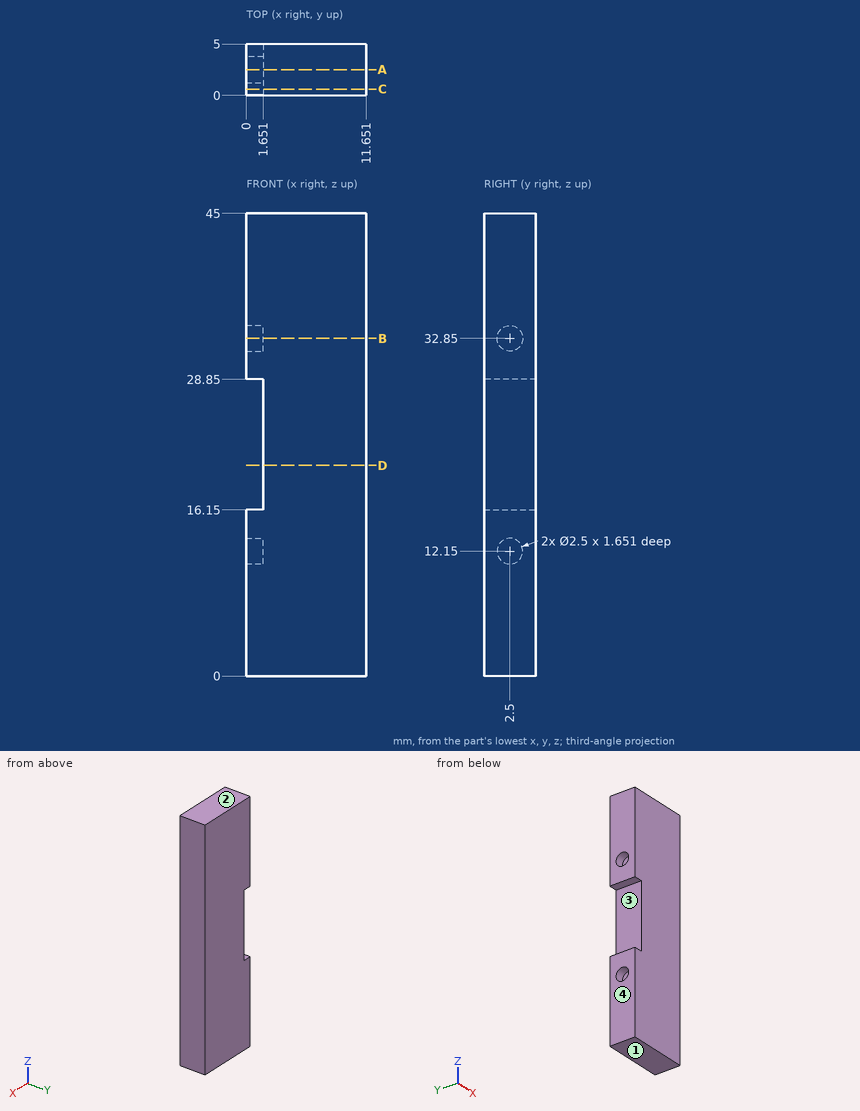
The drawing under review shows one solid part. Ordinate dimensions are in mm from its lowest x, y, z. Give positions to 0.01 mm unless a question says otherwise; leave off trailing zeros. Order: outer loops, then holes, each group sorted by start corner. A loop starts at its lowest first (then second) coordinate and runs counter-clockwise, first axis right, second up. Notation, with made-up numbers: (43, -15.5) -> (87, -15.5) arc R24 cw to (87, 4.5) -> close; hole circle Ø4 at (-25.75, -37). An arc over 180 degrees is marked (long way). Write item = value, one per line. Start each with the question number.
(1) We need section D-D on z = 20.5. Write out the cut boundary in (x, y).
(2) We need section B-B on z = 32.85. Write out the cut boundary in (x, y).
(3) To check wall thickness, follow line 1 along Y through (x, z) = (1.05, 32.85); line 2 along Z through (x, y) = (1, 2.5); line 3 along X through (y, z) = (4.05, 24). State the ranges of each line that lie inside material, in increasing order.
(4) For pin 1 (2 mm diameter, centred on y = 2.5, z = 12.15, fed in from -X), flat-tipped, find the tip position at first contact; note if it passes through.
(5) We need section C-C on y = 0.6. Write out the cut boundary in (x, z).
(6) Mouldability with a two-part tool opening along Z and no side actions: class the marked faces 1, 2, 3 and 4 as +Z half, -Z half, draft (parallel to the pull), parting line (faces both ways), or undercut.
(7) We need section A-A on y = 2.5. Write out the cut boundary in (x, z), plus the area to 3 significant figures.
Numbers:
q1.outline = (1.65, 0) -> (11.65, 0) -> (11.65, 5) -> (1.65, 5) -> close
q2.outline = (0, 0) -> (11.65, 0) -> (11.65, 5) -> (0, 5) -> (0, 3.75) -> (1.65, 3.75) -> (1.65, 1.25) -> (0, 1.25) -> close
q3.line_1 = 0 to 1.25, 3.75 to 5
q3.line_2 = 0 to 10.9, 13.4 to 16.15, 28.85 to 31.6, 34.1 to 45
q3.line_3 = 1.65 to 11.65
q4.pin_1 = 1.65
q5.outline = (0, 0) -> (11.65, 0) -> (11.65, 45) -> (0, 45) -> (0, 28.85) -> (1.65, 28.85) -> (1.65, 16.15) -> (0, 16.15) -> close
q6.face_1 = -Z half
q6.face_2 = +Z half
q6.face_3 = undercut
q6.face_4 = draft
q7.outline = (0, 0) -> (11.65, 0) -> (11.65, 45) -> (0, 45) -> (0, 34.1) -> (1.65, 34.1) -> (1.65, 31.6) -> (0, 31.6) -> (0, 28.85) -> (1.65, 28.85) -> (1.65, 16.15) -> (0, 16.15) -> (0, 13.4) -> (1.65, 13.4) -> (1.65, 10.9) -> (0, 10.9) -> close
q7.area = 495 mm^2
